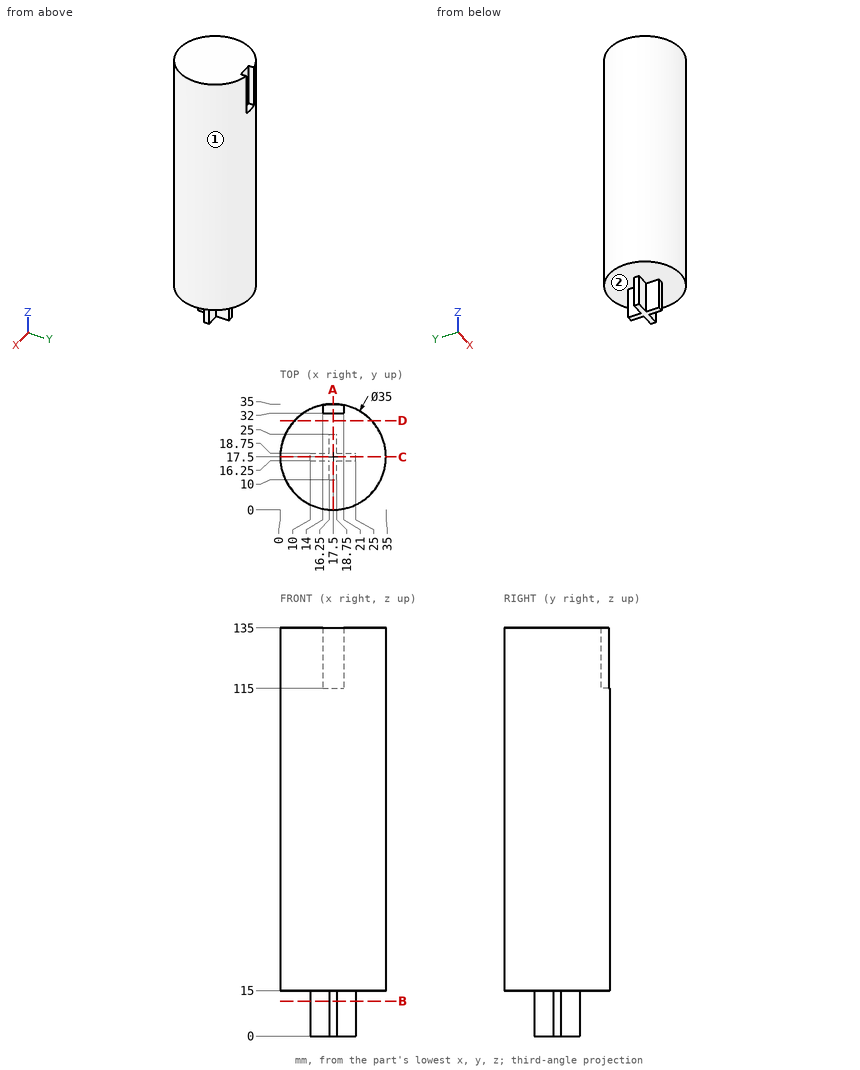
Input: dimensioned drawing with shaded views. Units: mm. Origin: part minimum x, y, z. Give positions to 0.01 mm unless a question says otherwise; leave off trailing zeros. Write each loop counter-clockwise with the first axis right and the second up, starting at its lowest first coordinate (ties: lowest second). Pieces come first, ordered by that corner, then holes.
Q1. First-contact query: P1, Ø3, axis at y = 18, z = 5.5, coming from the +X side; P2, Ø12, axis at x = 4, z = 37.5, coming from the -Y side; P3, Ø4, axis at x = 3.5, y = 20.5, coming from the -Z side. Flat tips, straight axial feed; report the tip coordinate or a pass-through.
Q2. Section C-C, the plane y = 17.5. Output: boundary loops of the cut face in (x, z), plus the area to 4 significant figures.
Q3. Material intervals for probe 1 along Z at (x, y) = (2.5, 26); probe 2 along Z at (x, y) = (14.5, 32.5); probe 3 along Y at (x, z) = (18, 84), sorted ascending.
Q4. Pull-direction query (X, two-part tool) for the marked faces 1 and 2; classes: pulls with the +X half, pulls with the -X half, needs draft (parallel to the pull), parting line crosses it, or undercut.
Q5. Section D-D, the plane y = 29.5. Output: boundary loops of the cut face in (x, z).
Q6. Section A-A, the plane x = 17.5. Output: boundary loops of the cut face in (y, z), plus the area to 4 significant figures.
Q7. Section B-B, the plane z = 11.5. Output: boundary loops of the cut face in (x, y).
Filled in:
1. P1: stops at x = 25
1. P2: stops at y = 1.69
1. P3: stops at z = 15
2. outline: (0, 15) - (10, 15) - (10, 0) - (25, 0) - (25, 15) - (35, 15) - (35, 135) - (0, 135) - close
2. area: 4,425 mm2
3. probe 1: z = 15 to 135
3. probe 2: z = 15 to 115
3. probe 3: y = 0.01 to 34.99
4. face 1: parting line crosses it
4. face 2: needs draft
5. outline: (4.76, 15) - (30.24, 15) - (30.24, 135) - (4.76, 135) - close
6. outline: (0, 15) - (10, 15) - (10, 0) - (25, 0) - (25, 15) - (35, 15) - (35, 115) - (32, 115) - (32, 135) - (0, 135) - close
6. area: 4,365 mm2
7. outline: (10, 16.25) - (16.25, 16.25) - (16.25, 10) - (18.75, 10) - (18.75, 16.25) - (25, 16.25) - (25, 18.75) - (18.75, 18.75) - (18.75, 25) - (16.25, 25) - (16.25, 18.75) - (10, 18.75) - close
